Input: part model. Units: mm. Frame: model coordinates. Face numbers are marked on the shaded views. A direction names the side the tool comes from. Round coordinates to 2 decimals unless told otherwise and drop trailing zeros. Order: outer loops, then holes, each group sorted by start corner. A loop starts at its lowest first (then second) coordinate and runs counter-clockwise, first axis right, second up. Notation, with made-up numbers: M 53.25,-15.5 L 84.25,-15.5 A24 cw 84.25,9.5 Z; hole C -29.5,79 d7. An arc over 180 degrees is marked long. One line per question, with ' | ' between items.
```python
from build123d import *

# Parameters (mm, degrees)
BOSS_EXTRUDE1_DEPTH = 75
SKETCH2_R           = 6
CUT_EXTRUDE1_DEPTH  = 96.315266353
BOSS_EXTRUDE2_DEPTH = 6
SKETCH4_R           = 18
BOSS_EXTRUDE3_DEPTH = 25
SKETCH5_R           = 11
CUT_EXTRUDE2_DEPTH  = 154.355795456


with BuildPart() as part:
    # Sketch1 → Boss-Extrude1 (new body)
    with BuildSketch(Plane.XY):
        Polygon((0, 0), (12, 0), (12, 6), (44, 6), (44, 0), (56, 0), (56, 18), (0, 18), align=None)
    extrude(amount=-BOSS_EXTRUDE1_DEPTH)

    # Sketch2 → Cut-Extrude1 (cut, through all)
    with BuildSketch(Plane(origin=(0, 18, 0), x_dir=(1, 0, 0), z_dir=(0, 1, 0))):
        with Locations(Location((28, 15, 0), (0, 0, 180))):
            Circle(SKETCH2_R)
        with Locations(Location((28, 60, 0), (0, 0, 180))):
            Circle(SKETCH2_R)
    extrude(amount=-CUT_EXTRUDE1_DEPTH, mode=Mode.SUBTRACT)

    # Sketch3 → Boss-Extrude2 (add, symmetric)
    with BuildSketch(Plane.XY.offset(-37.5)):
        Polygon((0, 18), (64, 63), (100, 63), (100, 38), (82, 38), (56, 0), (56, 18), align=None)
    extrude(amount=BOSS_EXTRUDE2_DEPTH, both=True)

    # Sketch4 → Boss-Extrude3 (add)
    with BuildSketch(Plane(origin=(0, 63, 0), x_dir=(1, 0, 0), z_dir=(0, 1, 0))):
        with Locations((100, 37.5)):
            Circle(SKETCH4_R)
    extrude(amount=-BOSS_EXTRUDE3_DEPTH)

    # Sketch5 → Cut-Extrude2 (cut, through all)
    with BuildSketch(Plane(origin=(0, 63, 0), x_dir=(1, 0, 0), z_dir=(0, 1, 0))):
        with Locations(Location((100, 37.5, 0), (0, 0, 270))):
            Circle(SKETCH5_R)
    extrude(amount=-CUT_EXTRUDE2_DEPTH, mode=Mode.SUBTRACT)


solid = part.part
```
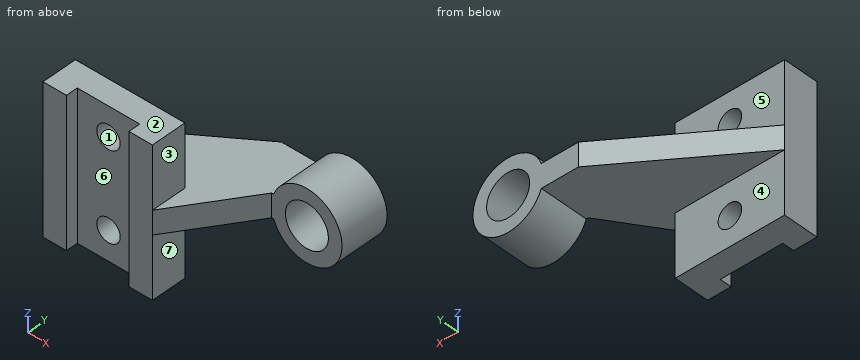
Item 1: Section query B-B, the plane z = -15. Return loops of the section in (x, y), plus the area to 3 significant figures.
Report:
outline: M 0,0 L 12,0 L 12,6 L 22,6 L 22,18 L 0,18 Z; M 34,6 L 44,6 L 44,0 L 56,0 L 56,18 L 34,18 Z | area: 672 mm²
Item 2: Section query D-D, the plane y = 11.5. Return loops of the section in (x, z).
Report:
outline: M 0,-75 L 56,-75 L 56,-43.5 L 63.87,-43.5 L 63.87,-31.5 L 56,-31.5 L 56,0 L 0,0 Z; hole C 28,-60 d12; hole C 28,-15 d12
Item 3: Section query C-C, the plane x = 28. Return loops of the section in (y, z), plus the area to 3 significant figures.
Report:
outline: M 6,-75 L 18,-75 L 18,-66 L 6,-66 Z; M 6,-54 L 18,-54 L 18,-43.5 L 37.69,-43.5 L 37.69,-31.5 L 18,-31.5 L 18,-21 L 6,-21 Z; M 6,-9 L 18,-9 L 18,0 L 6,0 Z | area: 848 mm²
Item 4: First-contact query: pin 1 (1.5 mm diameter, centred on x = 50.5, y = 26.5, fed in from +Z); pin 2 (9 mm diameter, centred on y = 10, z = -61, fed in from +X); pin 3 (19 mm diameter, centred on x = 28, z = -60, fed in from -Y). Flat tips, straight axial feed; report the tip coordinate or a pass-through.
Report:
pin 1: z = -31.5 | pin 2: x = 56 | pin 3: y = 6
Item 5: Mould query, pull axis Z, two halves, no side actions, for the marked faces 1, 2 and 3. Classes: +Z half, -Z half, draft (parallel to the pull), parting line (faces both ways), or undercut.
Report:
face 1: undercut | face 2: +Z half | face 3: draft
Item 6: Section query A-A, the plane x = 100. Return loops of the section in (y, z).
Report:
outline: M 38,-55.5 L 63,-55.5 L 63,-48.5 L 38,-48.5 Z; M 38,-26.5 L 63,-26.5 L 63,-19.5 L 38,-19.5 Z
Item 7: Access query for the marked faces 4, 5, 6 and 7. Directions: +Z, -Z, +X, -X, +Y, -Y. A direction counts if a zero-diameter tool reaches every point of the face in a straight line with its end or side. Return the directions, or none.
Report:
face 4: -Z, +X, -X, +Y | face 5: +Z, +X, -X, +Y | face 6: +Z, -Z, -Y | face 7: -Z, +X, +Y, -Y
Item 8: Line query: line 1 along Z through (x, y) = (28, 14.5); line 2 along Z through (x, y) = (67, 33); line 3 along Y through (x, z) = (9, -58). Output: solid intervals per line, ascending. Write a range as from..to.
Report:
line 1: -75..-66, -54..-21, -9..0 | line 2: -43.5..-31.5 | line 3: 0..18
